Check sheet for the modelled part. Datum: model origin and axes. Units: mm. A direction names the side the tool comes from. Round coordinates to 2 decimals unless told otherwise and drop trailing zeros. One line per item, written item: value. Start each with the question number.
```python
from build123d import *

# Parameters (mm, degrees)
F0_W      = 533.4
F0_H      = 863.6
F1_DEPTH  = 2.54
F2_W      = 533.4
F2_H      = 863.6
F2_W_2    = 508
F2_H_2    = 838.2
F3_DEPTH  = 254
F4_W      = 25.4
F4_H      = 406.4
F4_H_2    = 25.4
F5_DEPTH  = 254
F6_W      = 76.2
F6_H      = 190.5
F7_DEPTH  = 25.4
F8_W      = 76.2
F8_H      = 304.8
F9_DEPTH  = 25.4
F10_W     = 76.2
F10_H     = 279.4
F11_DEPTH = 25.4
F12_W     = 76.2
F12_H     = 254
F13_DEPTH = 25.4
F14_W     = 76.2
F14_H     = 228.6
F15_DEPTH = 25.4
F16_W     = 76.2
F16_H     = 203.2
F17_DEPTH = 25.4
F18_W     = 76.2
F18_H     = 177.8
F19_DEPTH = 25.4
F20_W     = 76.2
F20_H     = 152.4
F21_DEPTH = 25.4
F22_W     = 76.2
F22_H     = 127
F23_DEPTH = 25.4
F24_W     = 76.2
F24_H     = 101.6
F25_DEPTH = 25.4
F26_W     = 76.2
F26_H     = 76.2
F27_DEPTH = 25.4
F28_W     = 76.2
F28_H     = 190.5
F29_DEPTH = 25.4
F30_W     = 76.2
F30_H     = 190.5
F31_DEPTH = 25.4
F32_W     = 152.4
F32_H     = 190.5
F33_DEPTH = 25.4
F34_W     = 152.4
F34_H     = 190.5
F35_DEPTH = 25.4
F37_W     = 76.2
F37_H     = 76.2
F38_DEPTH = 25.4
F39_W     = 203.2
F39_H     = 127
F40_DEPTH = 25.4
F41_W     = 203.2
F41_H     = 127
F42_DEPTH = 25.4
F43_W     = 76.2
F43_H     = 190.5
F44_DEPTH = 25.4
F45_W     = 76.2
F45_H     = 190.5
F46_DEPTH = 25.4
F48_DEPTH = 12.7
F49_W     = 165.1
F49_H     = 127
F50_DEPTH = 25.4
F51_R     = 5.08
F52_DEPTH = 25.4
F53_W     = 190.5
F53_H     = 63.5
F54_DEPTH = 76.2
F55_W     = 165.1
F55_H     = 44.45
F56_DEPTH = 50.8
F57_W     = 127
F57_H     = 203.2
F57_W_2   = 76.2
F57_H_2   = 190.5
F58_DEPTH = 2.54
F60_DEPTH = 63.5
F61_W     = 50.8
F61_H     = 177.8
F62_DEPTH = 76.2
F64_DEPTH = 88.9
F65_W     = 50.8
F65_H     = 64.7032260895
F66_DEPTH = 177.8
F67_W     = 101.6
F67_H     = 203.2
F68_DEPTH = 88.9
F69_W     = 79.5584097505
F69_H     = 71.4426783538
F70_DEPTH = 203.2
F71_W     = 177.1770715714
F71_H     = 77.1189329839
F72_DEPTH = 101.6
F73_W     = 114.3
F73_H     = 81.28
F74_DEPTH = 12.7
F76_DEPTH = 76.2
F77_W     = 38.1
F77_H     = 45.72
F78_DEPTH = 50.8
F79_W     = 38.1
F79_H     = 8.466582
F79_H_2   = 6.773418
F80_DEPTH = 38.1


with BuildPart() as f1:
    # F0 (on Top) → F1 (new body)
    with BuildSketch(Plane.XY):
        Rectangle(F0_W, F0_H)
    extrude(amount=F1_DEPTH)

    # F2 (on face) → F3 (join)
    with BuildSketch(Plane.XY.offset(2.54)):
        Rectangle(F2_W, F2_H)
        Rectangle(F2_W_2, F2_H_2, mode=Mode.SUBTRACT)
    extrude(amount=F3_DEPTH)

    # F4 (on face) → F5 (join)
    with BuildSketch(Plane.XY.offset(2.54)):
        with Locations((38.1, -215.9)):
            Rectangle(F4_W, F4_H)
        with Locations((38.1, 0)):
            Rectangle(F4_W, F4_H_2)
        Polygon((254, 12.7), (50.8, 12.7), (50.8, -12.7), (254, -12.7), (254, 0), align=None)
        Polygon((25.4, -12.7), (25.4, 12.7), (-254, 12.7), (-254, 0), (-254, -12.7), align=None)
        with Locations((38.1, 215.9)):
            Rectangle(F4_W, F4_H)
    extrude(amount=F5_DEPTH)

    # F6 (on face) → F7 (cut)
    with BuildSketch(Plane.XZ.offset(431.8)):
        with Locations((177.8, 97.79)):
            Rectangle(F6_W, F6_H)
    extrude(amount=-F7_DEPTH, mode=Mode.SUBTRACT)

    # F8 (on face) → F9 (join)
    with BuildSketch(Plane.XY.offset(2.54)):
        with Locations((215.9, -165.1)):
            Rectangle(F8_W, F8_H)
    extrude(amount=F9_DEPTH)

    # F10 (on face) → F11 (join)
    with BuildSketch(Plane.XY.offset(27.94)):
        with Locations((215.9, -152.4)):
            Rectangle(F10_W, F10_H)
    extrude(amount=F11_DEPTH)

    # F12 (on face) → F13 (join)
    with BuildSketch(Plane.XY.offset(53.34)):
        with Locations((215.9, -139.7)):
            Rectangle(F12_W, F12_H)
    extrude(amount=F13_DEPTH)

    # F14 (on face) → F15 (join)
    with BuildSketch(Plane.XY.offset(78.74)):
        with Locations((215.9, -127)):
            Rectangle(F14_W, F14_H)
    extrude(amount=F15_DEPTH)

    # F16 (on face) → F17 (join)
    with BuildSketch(Plane.XY.offset(104.14)):
        with Locations((215.9, -114.3)):
            Rectangle(F16_W, F16_H)
    extrude(amount=F17_DEPTH)

    # F18 (on face) → F19 (join)
    with BuildSketch(Plane.XY.offset(129.54)):
        with Locations((215.9, -101.6)):
            Rectangle(F18_W, F18_H)
    extrude(amount=F19_DEPTH)

    # F20 (on face) → F21 (join)
    with BuildSketch(Plane.XY.offset(154.94)):
        with Locations((215.9, -88.9)):
            Rectangle(F20_W, F20_H)
    extrude(amount=F21_DEPTH)

    # F22 (on face) → F23 (join)
    with BuildSketch(Plane.XY.offset(180.34)):
        with Locations((215.9, -76.2)):
            Rectangle(F22_W, F22_H)
    extrude(amount=F23_DEPTH)

    # F24 (on face) → F25 (join)
    with BuildSketch(Plane.XY.offset(205.74)):
        with Locations((215.9, -63.5)):
            Rectangle(F24_W, F24_H)
    extrude(amount=F25_DEPTH)

    # F26 (on face) → F27 (join)
    with BuildSketch(Plane.XY.offset(231.14)):
        with Locations((215.9, -50.8)):
            Rectangle(F26_W, F26_H)
    extrude(amount=F27_DEPTH)

    # F28 (on face) → F29 (cut)
    with BuildSketch(Plane.XZ.offset(12.7)):
        with Locations((115.6540173054, 97.79)):
            Rectangle(F28_W, F28_H)
    extrude(amount=-F29_DEPTH, mode=Mode.SUBTRACT)

    # F30 (on face) → F31 (cut)
    with BuildSketch(Plane.YZ.offset(50.8)):
        with Locations((72.8943343222, 97.79)):
            Rectangle(F30_W, F30_H)
    extrude(amount=-F31_DEPTH, mode=Mode.SUBTRACT)

    # F32 (on face) → F33 (cut)
    with BuildSketch(Plane(origin=(0, 12.7, 0), x_dir=(-1, 0, 0), z_dir=(0, 1, 0))):
        with Locations((114.3, 97.79)):
            Rectangle(F32_W, F32_H)
    extrude(amount=-F33_DEPTH, mode=Mode.SUBTRACT)

    # F34 (on face) → F35 (cut)
    with BuildSketch(Plane(origin=(25.4, 0, 0), x_dir=(0, -1, 0), z_dir=(-1, 0, 0))):
        with Locations((279.4, 97.79)):
            Rectangle(F34_W, F34_H)
    extrude(amount=-F35_DEPTH, mode=Mode.SUBTRACT)

    # F37 (on face) → F38 (cut)
    with BuildSketch(Plane.YZ.offset(266.7)):
        with Locations((-335.3340667725, 185.5564373493)):
            Rectangle(F37_W, F37_H)
    extrude(amount=-F38_DEPTH, mode=Mode.SUBTRACT)

    # F39 (on face) → F40 (cut)
    with BuildSketch(Plane.XZ.offset(431.8)):
        with Locations((-114.3, 145.4548070431)):
            Rectangle(F39_W, F39_H)
    extrude(amount=-F40_DEPTH, mode=Mode.SUBTRACT)

    # F41 (on face) → F42 (cut)
    with BuildSketch(Plane(origin=(0, 431.8, 0), x_dir=(-1, 0, 0), z_dir=(0, 1, 0))):
        with Locations((114.3, 145.4548070431)):
            Rectangle(F41_W, F41_H)
    extrude(amount=-F42_DEPTH, mode=Mode.SUBTRACT)

    # F43 (on face) → F44 (cut)
    with BuildSketch(Plane(origin=(0, 431.8, 0), x_dir=(-1, 0, 0), z_dir=(0, 1, 0))):
        with Locations((-177.8, 97.79)):
            Rectangle(F43_W, F43_H)
    extrude(amount=-F44_DEPTH, mode=Mode.SUBTRACT)

    # F45 (on face) → F46 (cut)
    with BuildSketch(Plane(origin=(0, 12.7, 0), x_dir=(-1, 0, 0), z_dir=(0, 1, 0))):
        with Locations((-206.7097020388, 97.79)):
            Rectangle(F45_W, F45_H)
    extrude(amount=-F46_DEPTH, mode=Mode.SUBTRACT)

    # F47 (on face) → F48 (join)
    with BuildSketch(Plane(origin=(177.8, 0, 0), x_dir=(0, -1, 0), z_dir=(-1, 0, 0))):
        Polygon((88.9, 231.14), (88.9, 256.54), (12.7, 256.54), (12.7, 193.04), (12.7, 2.54), (317.5, 2.54), (317.5, 27.94), (292.1, 27.94), (292.1, 53.34), (266.7, 53.34), (266.7, 78.74), (241.3, 78.74), (241.3, 104.14), (215.9, 104.14), (215.9, 129.54), (190.5, 129.54), (190.5, 154.94), (165.1, 154.94), (165.1, 180.34), (139.7, 180.34), (139.7, 205.74), (114.3, 205.74), (114.3, 231.14), align=None)
    extrude(amount=F48_DEPTH)

    # F49 (on face) → F50 (cut)
    with BuildSketch(Plane(origin=(254, 0, 0), x_dir=(0, -1, 0), z_dir=(-1, 0, 0))):
        with Locations((-242.1909462929, 142.24)):
            Rectangle(F49_W, F49_H)
    extrude(amount=-F50_DEPTH, mode=Mode.SUBTRACT)

    # F51 (on face) → F52 (cut)
    with BuildSketch(Plane.XY.offset(256.54)):
        with Locations((259.08, -424.18)):
            Circle(F51_R)
        with Locations((-259.08, -424.18)):
            Circle(F51_R)
        with Locations((-259.08, 424.18)):
            Circle(F51_R)
        with Locations((259.08, 424.18)):
            Circle(F51_R)
    extrude(amount=-F52_DEPTH, mode=Mode.SUBTRACT)

    # F53 (on face) → F54 (join)
    with BuildSketch(Plane.XY.offset(2.54)):
        with Locations((-114.1317740679, -377.8158957958)):
            Rectangle(F53_W, F53_H)
    extrude(amount=F54_DEPTH)

    # F55 (on face) → F56 (cut)
    with BuildSketch(Plane.XY.offset(78.74)):
        with Locations((-114.1317740679, -368.2908957958)):
            Rectangle(F55_W, F55_H)
    extrude(amount=-F56_DEPTH, mode=Mode.SUBTRACT)

    # F57 (on face) → F58 (join)
    with BuildSketch(Plane.XY.offset(2.54)):
        with Locations((-114.1317740679, -203.2)):
            Rectangle(F57_W, F57_H)
        with Locations((107.7413304009, -203.2)):
            Rectangle(F57_W_2, F57_H_2)
    extrude(amount=F58_DEPTH)

    # F59 (on face) → F60 (join)
    with BuildSketch(Plane.XY.offset(2.54)):
        Polygon((215.9, 419.1), (197.4212676287, 419.1), (197.4212676287, 114.3), (254, 114.3), (254, 419.1), align=None)
    extrude(amount=F60_DEPTH)

    # F61 (on face) → F62 (join)
    with BuildSketch(Plane.XY.offset(2.54)):
        with Locations((76.2, 330.2)):
            Rectangle(F61_W, F61_H)
    extrude(amount=F62_DEPTH)

    # F63 (on face) → F64 (join)
    with BuildSketch(Plane.XY.offset(2.54)):
        Polygon((121.7336058617, 241.3), (101.6, 241.3), (50.8, 241.3), (50.8, 175.8374124765), (101.6, 175.8374124765), (121.7336058617, 175.8374124765), align=None)
    extrude(amount=F64_DEPTH)

    # F65 (on face) → F66 (join)
    with BuildSketch(Plane.XY.offset(2.54)):
        with Locations((76.2, 143.4857994318)):
            Rectangle(F65_W, F65_H)
    extrude(amount=F66_DEPTH)

    # F67 (on face) → F68 (join)
    with BuildSketch(Plane.XY.offset(2.54)):
        with Locations((-114.3, 215.9)):
            Rectangle(F67_W, F67_H)
    extrude(amount=F68_DEPTH)

    # F69 (on face) → F70 (cut)
    with BuildSketch(Plane.XZ.offset(-114.3)):
        with Locations((-113.5888062418, 38.2613391769)):
            Rectangle(F69_W, F69_H)
    extrude(amount=-F70_DEPTH, mode=Mode.SUBTRACT)

    # F71 (on face) → F72 (cut)
    with BuildSketch(Plane.YZ.offset(-63.5)):
        with Locations((216.2962853909, 41.0994664919)):
            Rectangle(F71_W, F71_H)
    extrude(amount=-F72_DEPTH, mode=Mode.SUBTRACT)

    # F73 (on face) → F74 (join)
    with BuildSketch(Plane.YZ.offset(-254)):
        with Locations((-237.8303322554, 178.4867082977)):
            Rectangle(F73_W, F73_H)
    extrude(amount=F74_DEPTH)

    # F75 (on face) → F76 (join)
    with BuildSketch(Plane.XY.offset(2.54)):
        Polygon((-46.28226161, -88.5335505009), (14.6819874644, -88.5335505009), (14.67773839, -27.5735505009), (-46.28226161, -27.5735505009), align=None)
    extrude(amount=F76_DEPTH)

    # F77 (on face) → F78 (cut)
    with BuildSketch(Plane.XY.offset(78.74)):
        with Locations((-27.23226161, -58.9001325009)):
            Rectangle(F77_W, F77_H)
    extrude(amount=-F78_DEPTH, mode=Mode.SUBTRACT)

    # F79 (on face) → F80 (cut)
    with BuildSketch(Plane.XY.offset(78.74)):
        with Locations((-27.23226161, -31.8068415009)):
            Rectangle(F79_W, F79_H)
        with Locations((-27.23226161, -85.1468415009)):
            Rectangle(F79_W, F79_H_2)
    extrude(amount=-F80_DEPTH, mode=Mode.SUBTRACT)


solid = f1.part
```
1. Depth check by flat-ended pin: pin 1 Ø12 at (x, y) = (-75.5, -108) entering from +Z; pin 2 Ø3 at (x, y) = (-259.5, 426) entering from +Z; pin 3 Ø6 at (y, z) = (257, 130.5) entering from +X. Enter the tip coordinate at first touch or a pass-through.
2. Access from +Z, -Z, +X, -X, +Y, -Y to the whole of each face (thin tool, end or side, straight path). Record for faces 1 (the face through (210, -203, 129.54)), 2 (the face through (-110, 304.885, 75)).
3. Release check for a two-part mould opening along Y. For faces 3 (the face through (210, -139.7, 193)), 4 (the face through (197.421, 269, 34)) record: +Y half, -Y half, draft (parallel to the pull), parting line (faces both ways), or undercut.
4. Material ranges on probe 1 along Y at (x, z) = (-226, 120); probe 2 along X at (y, z) = (-424.18, 244.25); probe 3 along Y at (x, z) = (259, 241), recorded low to high.
Working result:
1. pin 1: stops at z = 5.08
1. pin 2: stops at z = 231.14
1. pin 3: stops at x = 50.8
2. face 1: +Z
2. face 2: none
3. face 3: undercut
3. face 4: draft
4. probe 1: y = -431.8 to -419.1, -12.7 to 12.7, 419.1 to 431.8
4. probe 2: x = -266.7 to -264.16, -254 to 254, 264.16 to 266.7
4. probe 3: y = -431.8 to -429.26, -419.1 to 419.1, 429.26 to 431.8
